```python
from build123d import *

# Parameters (mm, degrees)
F1_R     = 53.975
F3_DEPTH = 10
F0_R     = 36.83
F4_DEPTH = 40
F5_T     = -2.54


with BuildPart() as f3:
    # F1 (on Top) → F3 (new body)
    with BuildSketch(Plane.XY):
        Circle(F1_R)
    extrude(amount=F3_DEPTH)

    # F0 (on Top) → F4 (join)
    with BuildSketch(Plane.XY):
        Circle(F0_R)
    extrude(amount=F4_DEPTH)

    # F5
    f5_openings = [f3.faces().sort_by_distance(p)[0] for p in [
        (0, 0, 40),
    ]]
    offset(amount=F5_T, openings=f5_openings, kind=Kind.INTERSECTION)


solid = f3.part
```
Source: CAD feature listing. Evaluate the final solid. Frame: model axes, mm. A direction names the side the tool comes from. Coordinates: 2 decimals unless noted, no trailing zeros. Write each loop counter-clockwise with the first axis right and the second up, starting at its lowest first coordinate (ties: lowest second). Pieces come first, ordered by that corner, then holes. Notation, with made-up numbers: M 33,-17 L 61,-17 A19 ccw 61,-6 Z; hole C 52,39 d4. An arc over 180 degrees is marked long. Answer as a JSON object with one key per item and string values.
1. Cut plane C-C on y = 46. Output: boundary loops of the cut face in (x, z), plus the area to 3 significant figures.
Evaluation:
{"outline": "M -28.24,0 L 28.24,0 L 28.24,10 L -28.24,10 Z; hole M -23.01,2.54 L 23.01,2.54 L 23.01,7.46 L -23.01,7.46 Z", "area": "338 mm^2"}
2. Access query for faces 4 (the cylindrical face through (-40.817, -31.297, 4.966)), 5 (the flat face through (-13, -35, 10)), 6 (the cylindrical face through (-39.78, 36.48, 4.93)). Directions: +Z, -Z, +X, -X, +Y, -Y. A direction counts if a zero-diameter tool reaches every point of the face in a straight line with its end or side. Return the directions, or none.
Evaluation:
{"face 4": "none", "face 5": "+Z", "face 6": "+Z, -Z"}
3. Cut plane B-B on z = 19. Output: boundary loops of the cut face in (x, y), plus the area to 3 significant figures.
Evaluation:
{"outline": "C 0,0 d73.66; hole C 0,0 d68.58", "area": "568 mm^2"}
4. Ray query, L1, parallel to Z at x = -1.5, y = -43.5; L2, parallel to X at y = 0, z = 25.5. Return the intervals inside material, ascending.
Evaluation:
{"L1": "0 to 2.54, 7.46 to 10", "L2": "-36.83 to -34.29, 34.29 to 36.83"}
5. Draft query along Z for faces 1 (the cylindrical face through (18.434, 28.913, 23.502)), 2 (the flat face through (-1, 1, 0)), 3 (the flat face through (11, -34, 7.46)). Return one class per face: released by +Z, released by -Z, zero draft, split by the parting line, or undercut.
Evaluation:
{"face 1": "zero draft", "face 2": "released by -Z", "face 3": "undercut"}
6. Cut plane A-A on y = 0. Output: boundary loops of the cut face in (x, z) (3 decimals), plus the area to 3 significant figures.
Evaluation:
{"outline": "M -53.975,0 L 53.975,0 L 53.975,10 L 36.83,10 L 36.83,40 L 34.29,40 L 34.29,7.46 L 51.435,7.46 L 51.435,2.54 L -51.435,2.54 L -51.435,7.46 L -34.29,7.46 L -34.29,40 L -36.83,40 L -36.83,10 L -53.975,10 Z", "area": "552 mm^2"}
7. Contact query for flat-ended pins moving along their axis: P1, Ø10, axis at y = 9, z = 4, coming from the +X side; P2, Ø1, axis at x = -12.5, y = -36.5, coming from the +Z side; P3, Ø4, axis at x = 28, z = 28, coming from the -Y side. Output: stop coordinate, or through.
Evaluation:
{"P1": "x = 53.83", "P2": "z = 10", "P3": "y = -26.09"}
